Design review of the part built by this model. Coordinates are the model's own, in mm. A direction names the side the tool comes from. Coordinates: 2 decimals unless noted, no trailing zeros. Write each loop counter-clockwise with the first axis right and the second up, starting at its lowest first coordinate (ties: lowest second). Pieces come first, ordered by that corner, then holes.
Q1. For L1, parallel to Y at x = 45, z = 4.5; L2, parallel to X at y = -123, z = 7.25; L3, parallel to X at y = -153.5, z = 3.5, list the stretches that pass through material, from the lowest coordinate up.
Q2. For pin 1 Ø8 at (x, y) = (23, -49.5) entering from -Z; pin 2 Ø5 at (y, z) = (-44.5, 6) entering from +X; pin 3 Ø5 at (x, z) = (7, 7) entering from +Y, all flat-tipped, find the tip position at first contact; note any pin that passes through.
Q3. The part is to be moulded in two halves that separate along Y. For faces 4 (the flat face through (15, -63, 0)), 5 (the flat face through (-9, 6, 5)), 6 (the flat face through (33.07, -90.05, 4.93)), say which applies: released by +Y, released by -Y, zero draft, split by the parting line, or undercut.
Q4. Take a section at A-A, the plane x = 30. Write out the cut boundary in (y, z), plus the area to 3 significant figures.
Q5. Take a section at D-D, the plane y = -135. Write out the cut boundary in (x, z), plus the area to 3 significant figures.
Q6. For faces 1 (the flat face through (43, -164, 5)), 2 (the flat face through (15, -63, 10)), 3 (the flat face through (-1, 3, 5)), list the 3-axis set-ups (+Z, -Z, +X, -X, +Y, -Y) from which the entire face can be reached by the end or side of a thin tool; tool diameter is ignored.
Q7. Take a section at C-C, the plane x = -8. Write out the cut boundary in (y, z), plus the area to 3 significant figures.
from build123d import *

# Parameters (mm, degrees)
F1_DEPTH = 10
F2_SIZE  = 1.99999
F3_SIZE  = 2.5


# Not quite as in the source:
# - a fillet or chamfer is up to 0.001 mm smaller than in the source, because OpenCascade refuses the exact size


with BuildPart() as f1:
    # F0 (on Top) → F1 (new body)
    with BuildSketch(Plane.XY):
        Polygon((35, 0), (0, 0), (-2, 6), (-17, 6), (-17, -14), (28, -14), (48, -14), (48, 6), (33, 6), (33, 1.5), (35, 1.5), align=None)
        Polygon((28, -14), (-17, -14), (28, -174), (48, -174), (48, -164), (38, -164), align=None)
    extrude(amount=F1_DEPTH)

    # F2 (size 2 in the source; OpenCascade refuses exactly that, so slightly less here)
    f2_edges = [f1.edges().sort_by_distance(p)[0] for p in [
        (33, 1.5, 5),
    ]]
    chamfer(f2_edges, length=F2_SIZE)

    # F3
    f3_edges = [f1.edges().sort_by_distance(p)[0] for p in [
        (33, 6, 5),
    ]]
    chamfer(f3_edges, length=F3_SIZE)


solid = f1.part
Responses:
1. L1: y = -174 to -164, -14 to 6
1. L2: x = 13.66 to 35.27
1. L3: x = 22.23 to 37.3
2. pin 1: stops at z = 0
2. pin 2: stops at x = 30.2
2. pin 3: stops at y = 0
3. face 4: zero draft
3. face 5: released by +Y
3. face 6: undercut
4. outline: (-174, 0) - (-44, 0) - (-44, 10) - (-174, 10) - close; (-14, 0) - (0, 0) - (0, 10) - (-14, 10) - close
4. area: 1,440 mm2
5. outline: (17.03, 0) - (36.07, 0) - (36.07, 10) - (17.03, 10) - close
5. area: 190 mm2
6. face 1: +Z, -Z, +X
6. face 2: +Z, +X, -X, +Y, -Y
6. face 3: +Z, -Z, +Y
7. outline: (-46, 0) - (6, 0) - (6, 10) - (-46, 10) - close
7. area: 520 mm2
